from build123d import *

# Parameters (mm, degrees)
BOX007_W     = 42
BOX007_H     = 50
BOX007_DEPTH = 15
BOX008_W     = 5
BOX008_H     = 36
BOX008_DEPTH = 15


with BuildPart() as cube006:
    # Box007 → Box007 (new body)
    with BuildSketch(Plane.XY):
        with Locations((21, 25)):
            Rectangle(BOX007_W, BOX007_H)
    extrude(amount=BOX007_DEPTH)


with BuildPart() as usb_fusion:
    # Box008 → Box008 (new body)
    with BuildSketch(Plane(origin=(42, 7, 0), x_dir=(1, 0, 0), z_dir=(0, 0, 1))):
        with Locations((2.5, 18)):
            Rectangle(BOX008_W, BOX008_H)
    extrude(amount=BOX008_DEPTH)

    # Fusion001: union Cube006
    add(cube006.part)


solid = usb_fusion.part
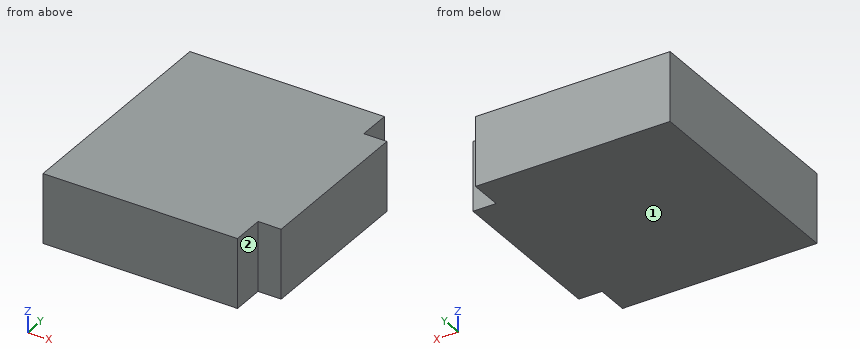
Can you work these out from the model? Positions are in its coordinate system, mm. Face numbers are marked on the shaded views. A direction names the side the tool comes from. Give positions to 0.01 mm unless a question says otherwise; leave off trailing zeros. Write each loop counter-clockwise with the first axis right and the second up, starting at its lowest first coordinate (ties: lowest second). Pieces come first, ordered by that corner, then holes. Notation, with made-up numbers: (-35, -10) -> (5, -10) arc R17 cw to (5, -3) -> close; hole circle Ø5 at (-26.75, 25.5). An arc over 180 degrees is marked (long way). Answer as a JSON object with one key per item and string values. Group by question number.
Item 1: For the marked faces 1 and 2, which set-ups out of +Z, -Z, +X, -X, +Y, -Y let a thin tool reach every point of the face, with its end or its side?
Item 2: Please list where these lines run through material, in increasing order: line 1 (X direction, y = 5, z = 9); line 2 (Y direction, x = 44, z = 2.5). Write a range as [from, to].
Item 3: I'm going to push flat-ended pins straight in: P1, Ø5.5, axis at y = 46, z = 8, coming from the +X side; P2, Ø1.5, axis at x = 45.5, z = 8, coming from the +Y side; P3, Ø5.5, axis at x = 45.5, z = 6.5, coming from the -Y side. Where does each tip first touch, or does it pass through?
Item 4: Suppose I cut it at A-A (z = 3.5). Please give me the cut outline in (x, y), plus the area to 3 significant figures.
Item 5: Suppose I cut it at B-B (y = 46.5). Please give me the cut outline in (x, z), plus the area to 3 significant figures.
Findings:
{
 "1": {"face 1": "-Z, +X, -X, +Y, -Y", "face 2": "+Z, -Z, +X, -Y"},
 "2": {"line 1": "x = [0, 42]", "line 2": "y = [7, 43]"},
 "3": {"P1": "stops at x = 42", "P2": "stops at y = 43", "P3": "stops at y = 7"},
 "4": {"outline": "(0, 0) -> (42, 0) -> (42, 7) -> (47, 7) -> (47, 43) -> (42, 43) -> (42, 50) -> (0, 50) -> close", "area": "2,280 mm²"},
 "5": {"outline": "(0, 0) -> (42, 0) -> (42, 15) -> (0, 15) -> close", "area": "630 mm²"}
}
